from build123d import *

# Parameters (mm, degrees)
F0_W      = 60.96
F0_H      = 86.36
F1_DEPTH  = 6.35
F1_FACE_W = 60.96
F1_FACE_H = 86.36
F6_DEPTH  = 86.361


with BuildPart() as f1:
    # F0 (on Front) → F1 (new body)
    with BuildSketch(Plane.XZ):
        Rectangle(F0_W, F0_H)
    extrude(amount=-F1_DEPTH)

    # F1_face (on face) → F4 section 0
    with BuildSketch(Plane(origin=(0, 6.35, 0), x_dir=(1, 0, 0), z_dir=(0, 1, 0)), mode=Mode.PRIVATE) as f4_s0:
        Rectangle(F1_FACE_W, F1_FACE_H)
    loft([f4_s0.sketch, Vertex(0, 50.8, 43.18)])

    # F5 (on face) → F6 (cut, through all)
    with BuildSketch(Plane.XY.offset(43.18)):
        Polygon((0, 39.571562), (-22.7805, 6.35), (22.7805, 6.35), align=None)
    extrude(amount=-F6_DEPTH, mode=Mode.SUBTRACT)


solid = f1.part
Model file for the job. Use its own axes, mm. A direction names the side the tool comes from. Give positions to 0.01 mm unless a question says otherwise; leave off trailing zeros. Loops run counter-clockwise (first coordinate to the right, second up) from the corner with the lowest first, then second, coordinate; pieces in that order, holes last.
1) Wall check: line 1 (Y direction, x = -2.5, z = -23); line 2 (Y direction, x = -20, z = 30); line 3 (X direction, y = 22.5, z = 23). Give the ranges that are in metal, low to high.
2) Pull direction Y, two halves, no side cores. Call faces 1 (the flat face through (14.08, 19.04, 10.2)), 2 (the flat face through (9.17, 27.03, -3)), 3 (the flat face through (30.48, 3, -1)): +Y half, -Y half, draft (parallel to the pull), parting line (faces both ways), or undercut.
3) Saw through at C-C (z = 26). Write the cut outline in (x, y).
4) Saw through at D-D (z = 8). Write the cut outline in (x, y), plus the area to 3 significant figures.
5) Saw through at A-A (x = -3). Write the cut outline in (y, z) (3 decimals), plus the area to 3 significant figures.
6) Flat gauge pins, fed straight in: pin 1 Ø1 at (x, z) = (-17, -27.5) entering from +Y; pin 2 Ø5 at (y, z) = (18, -1.5) entering from -X; pin 3 Ø1.5 at (y, z) = (8, 17.5) entering from -X. Where does each tip first touch, or does it go through?
7) Saw through at B-B (y = 7.5). Write the cut outline in (x, z), plus the area to 3 significant figures.
8) Tool access for faces 4 (the flat face through (0, 0, 1)), 5 (the flat face through (-13.762, 19.502, 10.2)): list every direction of +Z, -Z, +X, -X, +Y, -Y with a clear straight run to the whole face (end or side of a thin tool).
Answer block:
1. line 1: y = 0 to 6.35
1. line 2: y = 0 to 6.35, 10.4 to 21.63
1. line 3: x = -19.41 to -11.71, 11.71 to 19.41
2. face 1: undercut
2. face 2: +Y half
2. face 3: draft
3. outline: (-30.48, 0) - (30.48, 0) - (30.48, 6.35) - (6.06, 41.96) - (-6.06, 41.96) - (-30.48, 6.35) - close; hole (-22.78, 6.35) - (22.78, 6.35) - (0, 39.57) - close
4. outline: (-30.48, 0) - (30.48, 0) - (30.48, 6.35) - (12.42, 32.69) - (4.72, 32.69) - (22.78, 6.35) - (-22.78, 6.35) - (-4.72, 32.69) - (-12.42, 32.69) - (-30.48, 6.35) - close
4. area: 793 mm2
5. outline: (0, -43.18) - (6.35, -43.18) - (6.35, 43.18) - (0, 43.18) - close; (35.197, 12.865) - (46.425, 34.68) - (46.425, 43.18) - (35.197, 43.18) - close
5. area: 766 mm2
6. pin 1: stops at y = 14.68
6. pin 2: stops at x = -24.21
6. pin 3: stops at x = -29.86
7. outline: (-29.69, -40.95) - (-21.99, -40.95) - (-21.99, 43.18) - (-29.69, 43.18) - close; (21.99, -40.95) - (29.69, -40.95) - (29.69, 43.18) - (21.99, 43.18) - close
7. area: 1,300 mm2
8. face 4: +Z, -Z, +X, -X, -Y
8. face 5: +Z, -Z
